```python
from build123d import *

# Parameters (mm, degrees)
F1_DEPTH = 2540


with BuildPart() as f1:
    # F0 (on Front) → F1 (new body)
    with BuildSketch(Plane.XZ):
        with BuildLine():
            Line((-637.901507, -82.404926), (-129.901507, -82.404926))
            Line((-129.901507, -82.404926), (-129.901507, 44.595074))
            Line((-129.901507, 44.595074), (-295.001507, 44.595074))
            ThreePointArc((-295.001507, 44.595074), (-312.962019, 52.034562), (-320.401507, 69.995074))
            Line((-320.401507, 69.995074), (-320.401507, 654.195074))
            ThreePointArc((-320.401507, 654.195074), (-312.962019, 672.155587), (-295.001507, 679.595074))
            Line((-295.001507, 679.595074), (-129.901507, 679.595074))
            Line((-129.901507, 679.595074), (-129.901507, 806.595074))
            Line((-129.901507, 806.595074), (-637.901507, 806.595074))
            Line((-637.901507, 806.595074), (-637.901507, 679.595074))
            Line((-637.901507, 679.595074), (-472.801507, 679.595074))
            ThreePointArc((-472.801507, 679.595074), (-454.840994, 672.155587), (-447.401507, 654.195074))
            Line((-447.401507, 654.195074), (-447.401507, 69.995074))
            ThreePointArc((-447.401507, 69.995074), (-454.840994, 52.034562), (-472.801507, 44.595074))
            Line((-472.801507, 44.595074), (-637.901507, 44.595074))
            Line((-637.901507, 44.595074), (-637.901507, -82.404926))
        make_face()
    extrude(amount=F1_DEPTH)


solid = f1.part
```
Design review of the part built by this model. Coordinates are the model's own, in mm. A direction names the side the tool comes from. Give positions to 0.01 mm unless a question says otherwise; leave off trailing zeros. Write each loop counter-clockwise with the first axis right and the second up, starting at its lowest first coordinate (ties: lowest second). Pieces come first, ordered by that corner, then holes. Notation, with made-up numbers: (89, 50) -> (97, 50) arc R27 cw to (97, 88) -> close; hole circle Ø10 at (-33.75, -0.75). An arc over 180 degrees is marked (long way). Answer in a Markdown table with one row per item.
(1) To check wall thickness, follow probe 1 along Z at (x, y) = (-244, -241); probe 2 along X at (y, z) = (-1709, 587.5); probe 3 along Z at (x, y) = (-457, -1445). State the ranges of each line that lie inside material, in increasing order.
Results:
| item | result |
|---|---|
| probe 1 | -82.4 to 44.6, 679.6 to 806.6 |
| probe 2 | -447.4 to -320.4 |
| probe 3 | -82.4 to 50.11, 674.08 to 806.6 |
(2) Consider section C-C (z = 253.5). State the section outline as (x, y) points, then the cut area to 3 significant figures.
Results:
| item | result |
|---|---|
| outline | (-447.4, -2540) -> (-320.4, -2540) -> (-320.4, 0) -> (-447.4, 0) -> close |
| area | 323,000 mm2 |
(3) Mouldability with a two-part tool opening along Z and no side actions: class faces 1 (the flat face through (-557, -1252, 679.595)), 2 (the flat face through (-129.902, -1252, 742)), 3 (the flat face through (-387, -1252, -82.405)), 4 (the flat face through (-214, -1252, 679.595)) as +Z half, -Z half, draft (parallel to the pull), parting line (faces both ways), or undercut.
Results:
| item | result |
|---|---|
| face 1 | undercut |
| face 2 | draft |
| face 3 | -Z half |
| face 4 | undercut |
(4) Consider section B-B (y = -222). State the section outline as (x, z) points, then the cut area to 3 significant figures.
Results:
| item | result |
|---|---|
| outline | (-637.9, -82.4) -> (-129.9, -82.4) -> (-129.9, 44.6) -> (-295, 44.6) arc R25.4 cw to (-320.4, 70) -> (-320.4, 654.2) arc R25.4 cw to (-295, 679.6) -> (-129.9, 679.6) -> (-129.9, 806.6) -> (-637.9, 806.6) -> (-637.9, 679.6) -> (-472.8, 679.6) arc R25.4 cw to (-447.4, 654.2) -> (-447.4, 70) arc R25.4 cw to (-472.8, 44.6) -> (-637.9, 44.6) -> close |
| area | 210,000 mm2 |
(5) For faces 5 (the flat face through (-387, 0, 368)), 6 (the flat face through (-447.402, -1252, 366)), 7 (the flat face through (-320.402, -1252, 358)), list the 3-axis set-ups (+Z, -Z, +X, -X, +Y, -Y) from which the entire face can be reached by the end or side of a thin tool; tool diameter is ignored.
Results:
| item | result |
|---|---|
| face 5 | +Z, -Z, +X, -X, +Y |
| face 6 | -X, +Y, -Y |
| face 7 | +X, +Y, -Y |
(6) Consider section A-A (x = -593). State the section outline as (y, z) points.
Results:
| item | result |
|---|---|
| outline | (-2540, -82.4) -> (0, -82.4) -> (0, 44.6) -> (-2540, 44.6) -> close; (-2540, 679.6) -> (0, 679.6) -> (0, 806.6) -> (-2540, 806.6) -> close |
(7) Clearance check with flat-ended pins moving along their axes: pin 1 (3 mm diameter, centred on y = -1730.5, z = 167.5, fed in from +X); pin 2 (2 mm diameter, centred on y = -1707.5, z = 626.5, fed in from -X); pin 3 (4 mm diameter, centred on x = -375.5, z = 242.5, fed in from +Y). State where each tip first meets the part, or that it passes through.
Results:
| item | result |
|---|---|
| pin 1 | x = -320.4 |
| pin 2 | x = -447.4 |
| pin 3 | y = 0 |
